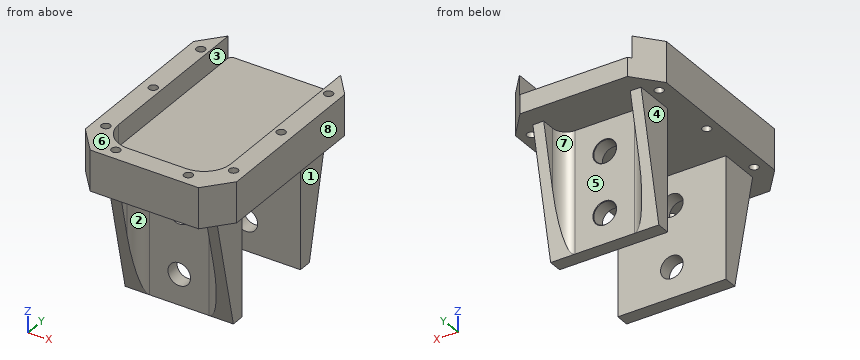
from build123d import *

# Parameters (mm, degrees)
SKETCH1_W                      = 35.56
SKETCH1_H                      = 50.8
BOSS_EXTRUDE1_DEPTH            = 9.525
SKETCH2_W                      = 26.4
SKETCH2_H                      = 46.22
CUT_EXTRUDE2_DEPTH             = 5.08
TAP_DRILL_FOR_M2_5X0_45_TAP1_D = 2.05
SKETCH13_W                     = 25.4
SKETCH13_H                     = 3.175
BOSS_EXTRUDE2_DEPTH            = 28.575
CUT_EXTRUDE3_DEPTH             = 73.778867812
FILLET1_R                      = 6.35
M5_CLEARANCE_HOLE1_D           = 5.3
M5_CLEARANCE_HOLE1_CSINK_D     = 5.55
M5_CLEARANCE_HOLE1_CSINK_ANGLE = 90
RIB7_REACH                     = 67.774
SKETCH14_WALL_W                = 162.819779212
SKETCH14_WALL_H                = 2.54
RIB8_START                     = -2.54
RIB8_DEPTH                     = 2.54
RIB9_REACH                     = 67.774
SKETCH17_WALL_W                = 162.819779212
SKETCH17_WALL_H                = 2.54
RIB10_START                    = -2.54
RIB10_DEPTH                    = 2.54
FILLET2_R                      = 3.175
FILLET3_R                      = 3.175


# Read off the part's stored shape, not the designer's step: Rib8, Rib10
with BuildPart() as part:
    # Sketch1 → Boss-Extrude1 (new body)
    with BuildSketch(Plane.XY):
        with Locations((-17.78, 25.4)):
            Rectangle(SKETCH1_W, SKETCH1_H)
    extrude(amount=BOSS_EXTRUDE1_DEPTH)

    # Sketch2 → Cut-Extrude2 (cut)
    with BuildSketch(Plane.XY.offset(9.525)):
        with Locations((-17.78, 27.69)):
            Rectangle(SKETCH2_W, SKETCH2_H)
    extrude(amount=-CUT_EXTRUDE2_DEPTH, mode=Mode.SUBTRACT)

    # Tap Drill for M2.5x0.45 Tap1 (through all)
    with Locations(Plane(origin=(0, 0, 0), x_dir=(-1, 0, 0), z_dir=(0, 0, -1))):
        with Locations((2.792369004, 43.087106138), (2.792369004, 26.092979092), (2.792369004, 9.105182099), (9.290740849, 2.822744672), (26.292369004, 2.787106138), (32.780032006, 9.105182099), (32.792369004, 26.087106138), (32.792369004, 43.087106138)):
            Hole(TAP_DRILL_FOR_M2_5X0_45_TAP1_D / 2)

    # Sketch13 → Boss-Extrude2 (add)
    with BuildSketch(Plane(origin=(0, 0, 0), x_dir=(-1, 0, 0), z_dir=(0, 0, -1))):
        with Locations((17.78, 38.091545037)):
            Rectangle(SKETCH13_W, SKETCH13_H)
        with Locations((17.78, 14.088545037)):
            Rectangle(SKETCH13_W, SKETCH13_H)
    extrude(amount=BOSS_EXTRUDE2_DEPTH)

    # Sketch8 → Cut-Extrude3 (cut, through all)
    with BuildSketch(Plane.XY.offset(9.525)):
        Polygon((-5.178964387, 50.8), (0, 44.591495864), (0, 50.8), align=None)
        Polygon((-35.56, 44.706622517), (-35.56, 50.8), (-30.402645731, 50.8), align=None)
        Polygon((-35.56, 5.970049098), (-35.56, 0), (-30.492594088, 0), align=None)
        Polygon((-5.092594088, -0.031324356), (0, 0), (0, 5.970049098), align=None)
    extrude(amount=-CUT_EXTRUDE3_DEPTH, mode=Mode.SUBTRACT)

    # Fillet1
    fillet1_edges = [part.edges().sort_by_distance(p)[0] for p in [
        (-30.98, 4.58, 6.985),
        (-4.58, 4.58, 6.985),
    ]]
    fillet(fillet1_edges, radius=FILLET1_R)

    # M5 Clearance Hole1 (through all)
    with Locations(Plane(origin=(-17.78, 39.679045037, -7.14375), x_dir=(0, 0, 1), z_dir=(0, 1, 0))):
        with Locations((0, 0), (-14.2875, 0)):
            CounterSinkHole(M5_CLEARANCE_HOLE1_D / 2, M5_CLEARANCE_HOLE1_CSINK_D / 2, counter_sink_angle=M5_CLEARANCE_HOLE1_CSINK_ANGLE)

    # Sketch14 wall → Rib7 (add, up to next)
    with BuildSketch(Plane(origin=(-30.48, 9.326045037, -14.2875), x_dir=(0, -0.216930457819, 0.976187060184), z_dir=(0, 0.976187060184, 0.216930457819)), mode=Mode.PRIVATE) as rib7_sk1:
        with Locations((0, 1.27)):
            Rectangle(SKETCH14_WALL_W, SKETCH14_WALL_H)
    rib7_tool1 = extrude(rib7_sk1.sketch, amount=RIB7_REACH, mode=Mode.PRIVATE) - part.part
    add(rib7_tool1.solids().sort_by_distance((-30.48, 9.326045037, -14.2875))[0])

    # Rib8 outline → Rib8 (add)
    with BuildSketch(Plane(origin=(-5.08, 0, 0), x_dir=(0, 0, -1), z_dir=(1, 0, 0)).offset(RIB8_START)):
        Polygon((0, 6.151045037), (28.575, 12.501045037), (0, 12.501045037), align=None)
    extrude(amount=RIB8_DEPTH)

    # Sketch17 wall → Rib9 (add, up to next)
    with BuildSketch(Plane(origin=(-5.08, 42.854045037, -14.2875), x_dir=(0, 0.216930457819, 0.976187060184), z_dir=(0, -0.976187060184, 0.216930457819)), mode=Mode.PRIVATE) as rib9_sk1:
        with Locations((0, 1.27)):
            Rectangle(SKETCH17_WALL_W, SKETCH17_WALL_H)
    rib9_tool1 = extrude(rib9_sk1.sketch, amount=RIB9_REACH, mode=Mode.PRIVATE) - part.part
    add(rib9_tool1.solids().sort_by_distance((-5.08, 42.854045037, -14.2875))[0])

    # Rib10 outline → Rib10 (add)
    with BuildSketch(Plane.ZY.offset(30.48).offset(RIB10_START)):
        Polygon((0, 46.029045037), (-28.575, 39.679045037), (0, 39.679045037), align=None)
    extrude(amount=RIB10_DEPTH)

    # Fillet2
    fillet2_edges = [part.edges().sort_by_distance(p)[0] for p in [
        (-27.94, 12.501045037, -14.2875),
        (-7.62, 12.501045037, -14.2875),
    ]]
    fillet(fillet2_edges, radius=FILLET2_R)

    # Fillet3
    fillet3_edges = [part.edges().sort_by_distance(p)[0] for p in [
        (-7.62, 39.679045037, -14.2875),
        (-27.94, 39.679045037, -14.2875),
    ]]
    fillet(fillet3_edges, radius=FILLET3_R)


solid = part.part
The listing builds one solid part. Answer for the finished solid, in the listing's coordinates (mm). Face numbers are marked on the shaded views. A direction names the side the tool comes from. Coordinates: 2 decimals unless noted, no trailing zeros. Loops run counter-clockwise (first coordinate to the right, second up) from the corner with the lowest first, then second, coordinate; pieces in that order, holes last.
1) Find section C-C on z = -16. Write down the section's boundary in (x, y) (3 decimals).
2) Flat-ended cylindrical pins translate along their axes: pin 1 Ø7 at (x, z) = (-17.78, -7.14) entering from +Y; pin 2 Ø3 at (x, y) = (-25, 30.5) entering from -Z; pin 3 Ø1.8 at (x, y) = (-32.78, 9.11) entering from -Z; pin 4 Ø10 at (x, y) = (-15.5, 41) entering from +Z (3 decimals). Find the tip coordinate at first contact, or state that the pin passes through.
3) A tool of negligible diameter and unlimited length cuts with its end or side. For the marked faces 1, 2, 3, 4 and 5, from which of +Z, -Z, +X, -X, +Y, -Y can it reach the whole face along a straight path? Write none if from no direction.
4) Find the intervals of material crossed by L1, parallel to Z at x = -17, y = 38 (3 decimals); L2, parallel to Y at x = -2, z = 6; L3, parallel to Y at x = -3, z = 1, in increasing order.
5) Find section D-D on x = -21.5. Write down the section's boundary in (y, z) (3 decimals).
6) Find section A-A on x = -17.78. Give the number of separate pieces and of enclosed holes in the cut face, then the cut area to 3 significant figures.
7) Find section B-B on y = 31.5. Write down the section's boundary in (x, z) (3 decimals).
8) Determine the mould class of the marked faces 6, 7 and 8 for opening direction X: pulls with the +X half, pulls with the -X half, needs draft (parallel to the pull), parting line crosses it, or undercut.
Values:
1. outline: (-30.48, 9.707) - (-27.917, 9.707) arc R3.175 cw to (-24.765, 12.501) - (-10.795, 12.501) arc R3.175 cw to (-7.643, 9.707) - (-5.08, 9.707) - (-5.08, 15.676) - (-30.48, 15.676) - close; (-30.48, 36.504) - (-5.08, 36.504) - (-5.08, 42.473) - (-7.643, 42.473) arc R3.175 cw to (-10.795, 39.679) - (-24.765, 39.679) arc R3.175 cw to (-27.917, 42.473) - (-30.48, 42.473) - close
2. pin 1: stops at y = 39.68
2. pin 2: stops at z = 0
2. pin 3: passes through
2. pin 4: stops at z = 4.445
3. face 1: -Z, +X, +Y, -Y
3. face 2: -Z, -Y
3. face 3: +Z, +Y
3. face 4: -Z, -X, +Y, -Y
3. face 5: -Z, +Y
4. L1: z = -28.575 to -23.964, -18.899 to -9.676, -4.611 to 4.445
4. L2: y = 3.61 to 8.45, 9.76 to 25.44, 26.74 to 42.44, 43.74 to 46.99
4. L3: y = 2.43 to 8.1, 10.11 to 25.09, 27.1 to 42.08, 44.09 to 48.19
5. outline: (0, 0) - (12.501, 0) - (12.501, -28.575) - (15.676, -28.575) - (15.676, 0) - (36.504, 0) - (36.504, -28.575) - (39.679, -28.575) - (39.679, 0) - (50.8, 0) - (50.8, 4.445) - (4.58, 4.445) - (4.58, 9.525) - (0, 9.525) - close
6. separate pieces: 5
6. enclosed holes: 0
6. area: 363 mm2
7. outline: (-35.56, 0) - (0, 0) - (0, 9.525) - (-4.58, 9.525) - (-4.58, 4.445) - (-30.98, 4.445) - (-30.98, 9.525) - (-35.56, 9.525) - close
8. face 6: needs draft
8. face 7: undercut
8. face 8: pulls with the +X half
